Read the model definition and answer for the solid it produces. Units are mm, in the model's axes. A direction names the side the tool comes from. Coordinates: 2 decimals unless noted, no trailing zeros. Loops run counter-clockwise (first coordinate to the right, second up) from the corner with the lowest first, then second, coordinate; pieces in that order, holes last.
from build123d import *

# Parameters (mm, degrees)
EXTRUDE_1_DEPTH                  = 10
FILLET_1_R                       = 2
PATTERN_CIRCULAR_2_COUNT         = 3
FILLET_1_OF_PATTERN_CIRCULAR_2_R = 2
CUT_EXTRUDE_START                = -15
SKETCH_3_R                       = 51
CUT_EXTRUDE_1_DEPTH              = 15
SKETCH_4_R                       = 62.618720145
SKETCH_4_R_2                     = 57
CUT_EXTRUDE_2_DEPTH              = 15
CHAMFER_1_SIZE                   = 2
FILLET_2_R                       = 5


with BuildPart() as part:
    # Эскиз1 → Повернуть1 (revolve)
    with BuildSketch(Plane(origin=(0, 0, 0), x_dir=(1, 0, 0), z_dir=(0, 1, 0))):
        Polygon((0, 0), (-54, 0), (-54, 145), (-51, 145), (-51, 3), (0, 3), align=None)
    revolve(axis=Axis((0, 0, -3), (0, 0, 1)))

    # Эскиз2 → Бобышка-Вытянуть1 (add)
    with BuildSketch(Plane(origin=(57, 0, 0), x_dir=(0, 0, -1), z_dir=(1, 0, 0))):
        Polygon((145, 14), (145, -14), (140, -14), (138.5, 11), (134, 11), (134, 14), align=None)
    extrude_1 = extrude(amount=-EXTRUDE_1_DEPTH)

    # Скругление1
    fillet_1_edges = [part.edges().sort_by_distance(p)[0] for p in [
        (54.576809621, -14, -140),
    ]]
    fillet(fillet_1_edges, radius=FILLET_1_R)

    # Круговой массив2: Бобышка-Вытянуть1 ×3 about axis
    pattern_circular_2_axis = Axis((0, 0, 0), (0, 0, 1))
    for i in range(1, PATTERN_CIRCULAR_2_COUNT):
        add(extrude_1.rotate(pattern_circular_2_axis, i * 360 / PATTERN_CIRCULAR_2_COUNT))

    # Скругление1 of Круговой массив2
    fillet_1_of_pattern_circular_2_edges = [part.edges().sort_by_distance(p)[0] for p in [
        (-15.164049157, 54.264903589, -140),
        (-39.412760463, -40.264903589, -140),
    ]]
    fillet(fillet_1_of_pattern_circular_2_edges, radius=FILLET_1_OF_PATTERN_CIRCULAR_2_R)

    # Эскиз3 → Вырез-Вытянуть1 (cut)
    with BuildSketch(Plane(origin=(0, 0, -145), x_dir=(-1, 0, 0), z_dir=(0, 0, -1)).offset(CUT_EXTRUDE_START)):
        Circle(SKETCH_3_R)
    extrude(amount=CUT_EXTRUDE_1_DEPTH, mode=Mode.SUBTRACT)

    # Эскиз4 → Вырез-Вытянуть2 (cut)
    with BuildSketch(Plane(origin=(0, 0, -145), x_dir=(-1, 0, 0), z_dir=(0, 0, -1))):
        Circle(SKETCH_4_R)
        Circle(SKETCH_4_R_2, mode=Mode.SUBTRACT)
    extrude(amount=-CUT_EXTRUDE_2_DEPTH, mode=Mode.SUBTRACT)

    # Фаска1
    chamfer_1_edges = [part.edges().sort_by_distance(p)[0] for p in [
        (54, 0, 0),
    ]]
    chamfer(chamfer_1_edges, length=CHAMFER_1_SIZE)

    # Скругление2
    fillet_2_edges = [part.edges().sort_by_distance(p)[0] for p in [
        (51, 0, -3),
    ]]
    fillet(fillet_2_edges, radius=FILLET_2_R)


solid = part.part
Q1. Straight lines are drawn through the part: probe 1 along Y at (x, z) = (0, -67); probe 2 along Z at (x, y) = (-19.5, 4.5). For each, find the intervals that lie inside material, in ascending order.
Findings below:
probe 1: y = -54 to -51, 51 to 54
probe 2: z = -3 to 0
Q2. Which of the six approach directions +Z, -Z, +X, -X, +Y, -Y give full straight-line access (tool end or side, diameter ignored) to faces 5 (the face through (-16, -53, -134)), 6 (the face through (11.706, 52.716, -74.501)), 7 (the face through (-38, 41, -134))?
Findings below:
face 5: +Z, -X, -Y
face 6: +Z
face 7: +Z, -X, +Y
Q3. A cutting plane is placed at C-C (z = -62). Give the vertices of the cut face in (x, y).
Findings below:
outline: circle Ø108 at (0, 0); hole circle Ø102 at (0, 0)
Q4. A cutting plane is placed at A-A (y = 0). Give the vertices of the cut face in (x, z), then the cut area to 3 significant figures.
Findings below:
outline: (-54, -145) - (-51, -145) - (-51, -8) arc R5 cw to (-46, -3) - (46, -3) arc R5 cw to (51, -8) - (51, -145) - (57, -145) - (57, -139.16) - (54, -139.16) - (54, -2) - (52, 0) - (-52, 0) - (-54, -2) - close
area: 1,200 mm2
Q5. A cutting plane is placed at B-B (x = 0). Give the vertices of the cut face in (y, z).
Findings below:
outline: (-54, -145) - (-51, -145) - (-51, -8) arc R5 cw to (-46, -3) - (46, -3) arc R5 cw to (51, -8) - (51, -145) - (54, -145) - (54, -2) - (52, 0) - (-52, 0) - (-54, -2) - close
Q6. Flat-ended cylindrical pins translate along their axes: pin 1 Ø3 at (x, y) = (24.5, -24) entering from -Z; pin 2 Ø1.5 at (x, y) = (54, 12) entering from +Z; pin 3 Ø2.5 at (x, z) = (54.5, -143.5) entering from -Y; pin 4 Ø10 at (x, y) = (-25.5, 24) entering from +Z. Find the tip coordinate at first contact, or state that the pin passes through.
Findings below:
pin 1: stops at z = -3
pin 2: stops at z = -134
pin 3: stops at y = -14
pin 4: stops at z = 0
Q7. Determine the mould class of faces 1 (the face through (-15.28, 53.41, -140.53)), 2 (the face through (57, 0, -142)), 3 (the face through (1, -1, -3)), 4 (the face through (11.056, 49.787, -75.541)) for opening direction Y: +Y half, -Y half, draft (parallel to the pull), parting line (faces both ways), or undercut.
Findings below:
face 1: +Y half
face 2: parting line
face 3: undercut
face 4: undercut
